Geometry: see drawing. Coordinates: mm, zero at the bounding-box minimum. Coordinates: 2 decimals unless noted, no trailing zeros. Write each loop counter-clockwise with the first axis right and the second up, starting at its lowest first coordinate (ties: lowest second). Pieces come first, ordered by that corner, then holes. Notation, with made-up numbers: M 24.5,53 L 37.5,53 A17 cw 37.5,63 Z; hole C 12,87 d2. An arc over 180 degrees is marked long. One line per item, written item: value. Start each with the question number.
Item 1: Cut plane B-B, the plane z = 12. Output: boundary loops of the cut face in (x, y).
Item 2: Pin query (flat end, axial travel): P1, Ø2, axis at x = 6.5, z = 6.5, coming from the +Y side. Return the tip coordinate at first contact, or that it passes through.
Item 3: Cut plane D-D, the plane z = 2.5. Output: boundary loops of the cut face in (x, y), then the cut area to 3 significant figures.
Item 4: Cut plane C-C, the plane y = 150. Output: boundary loops of the cut face in (x, z).
Item 5: Ray query, L1, parallel to Y at x = 4.5, z = 10; L2, parallel to Y at x = 2, z = 14.25; L3, parallel to Z at x = 3.25, y = 150. Return the intervals inside material, ascending. Write a range as from..to.
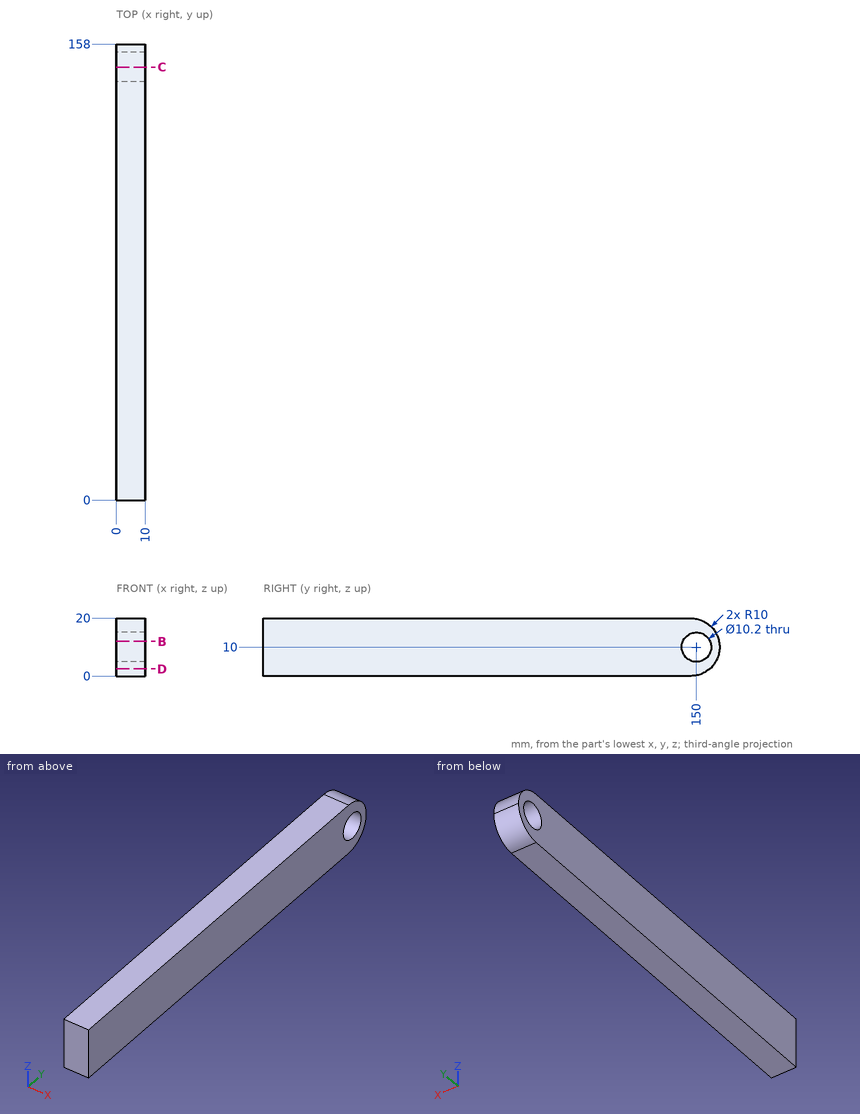
From the geometry:
1. outline: M 0,0 L 10,0 L 10,145.31 L 0,145.31 Z; M 0,154.69 L 10,154.69 L 10,157.8 L 0,157.8 Z
2. P1: stops at y = 157.68
3. outline: M 0,0 L 10,0 L 10,154.61 L 0,154.61 Z
3. area: 1,550 mm²
4. outline: M 0,0.2 L 10,0.2 L 10,4.9 L 0,4.9 Z; M 0,15.1 L 10,15.1 L 10,19.8 L 0,19.8 Z
5. L1: y = 0..144.9, 155.1..158
5. L2: y = 0..147.18, 152.82..157.05
5. L3: z = 0.2..4.9, 15.1..19.8
